Job drawing, mm, ordinate dimensions from the low corner. One solid piece. A direction names the side the tool comes from. Coordinates: 2 decimals unless noted, no trailing zeros. Write each loop counter-clockwise with the first axis right and the second up, starting at its lowest first coordinate (ties: lowest second). Pieces come first, ordered by that corner, then holes. Notation, with made-up numbers: (38.5, -24) - (85.5, -24) arc R19 cw to (85.5, -3) - close; hole circle Ø5 at (83, -24). An arc over 180 degrees is marked (long way). Put each result on its own line as item: value. Start each with the question number.
1. Drop flat-ended pins along their axis: P1, Ø2.5, axis at x = 51.5, y = 16.5, coming from the -Z side; P2, Ø11.5, axis at x = 30, y = 14, coming from the +Z side; P3, Ø6, axis at y = 17, z = 26, coming from the -X side; P4, Ø5, axis at x = 44.5, z = 26, coming from the +Y side. Give the stop position or say it passes through.
2. Saw through at B-B, the plane z = 16. Write the cut outline in (x, y).
3. Saw through at A-A, the plane x = 52.5. Write the cut outline in (y, z).
4. Drill centre lines: L1, parallel to Y at x = 52.5, z = 31; L2, parallel to X at y = 0.7, z = 16; L3, parallel to Y at x = 5.5, z = 30.95. Where is each one in solid material? Low to high. Write a range as from..to.
5. Saw through at D-D, the plane x = 39. Write the cut outline in (y, z).
6. Saw through at C-C, the plane y = 6.5. Write the cut outline in (x, z).
7. Which spindle directions (+Z, -Z, +X, -X, +Y, -Y) get a long thin tool onto all of the face, cutting with end or side? Do the marked faces 1 and 2. Say none if no direction does.
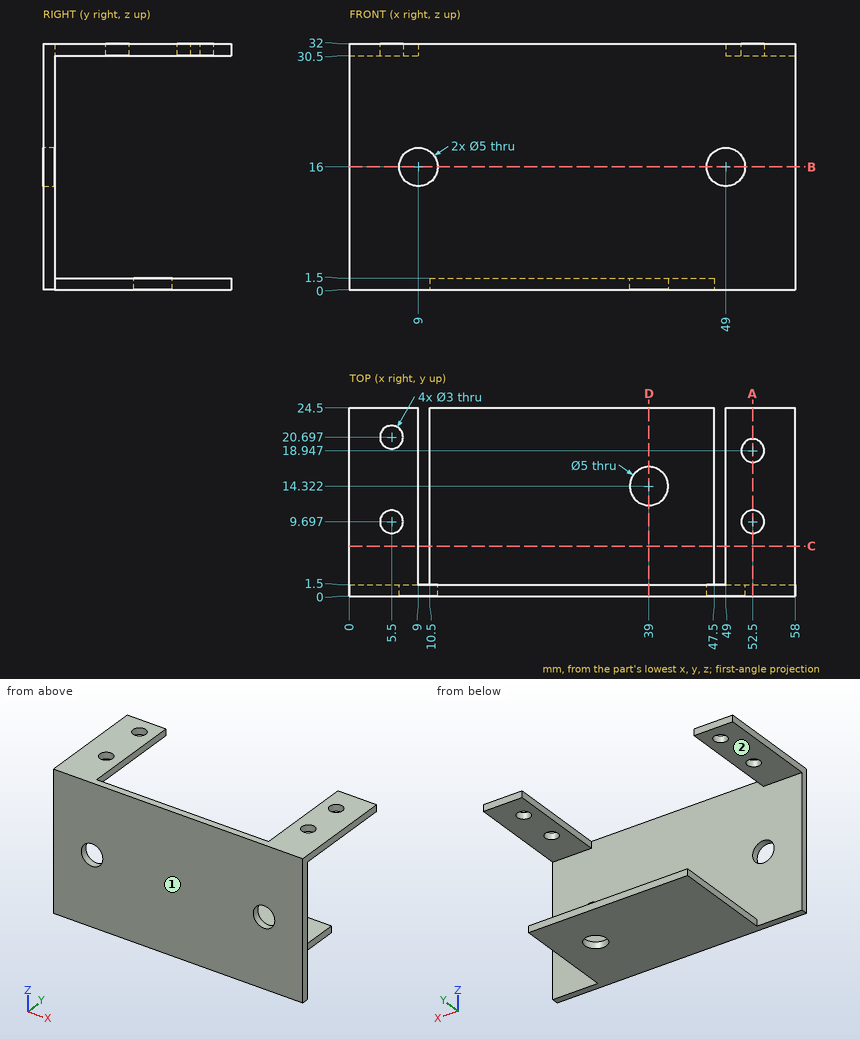
Final values:
1. P1: stops at z = 30.5
1. P2: stops at z = 1.5
1. P3: passes through
1. P4: stops at y = 1.5
2. outline: (0, 0) - (6.5, 0) - (6.5, 1.5) - (0, 1.5) - close; (11.5, 0) - (46.5, 0) - (46.5, 1.5) - (11.5, 1.5) - close; (51.5, 0) - (58, 0) - (58, 1.5) - (51.5, 1.5) - close
3. outline: (0, 0) - (1.5, 0) - (1.5, 30.5) - (8.2, 30.5) - (8.2, 32) - (0, 32) - close; (11.2, 30.5) - (17.45, 30.5) - (17.45, 32) - (11.2, 32) - close; (20.45, 30.5) - (24.5, 30.5) - (24.5, 32) - (20.45, 32) - close
4. L1: y = 0..8.2, 11.2..17.45, 20.45..24.5
4. L2: x = 0..6.5, 11.5..46.5, 51.5..58
4. L3: y = 0..8.2, 11.2..19.2, 22.2..24.5
5. outline: (0, 0) - (11.82, 0) - (11.82, 1.5) - (1.5, 1.5) - (1.5, 32) - (0, 32) - close; (16.82, 0) - (24.5, 0) - (24.5, 1.5) - (16.82, 1.5) - close
6. outline: (0, 30.5) - (9, 30.5) - (9, 32) - (0, 32) - close; (10.5, 0) - (47.5, 0) - (47.5, 1.5) - (10.5, 1.5) - close; (49, 30.5) - (58, 30.5) - (58, 32) - (49, 32) - close
7. face 1: +Z, -Z, +X, -X, -Y
7. face 2: -Z, +X, -X, +Y
